Answer from the drawing. Dimensions are ordinates in mm from the lowest x, y and z of the part. Round coordinates to 2 decimals unless told otherwise and drop trailing zeros. Loops run counter-clockwise (first coordinate to the right, second up) from the corner with the lowest first, then second, coordinate; pieces in that order, holes last. Notation, with made-up numbers: M 10.5,-26 L 59.5,-26 A23 cw 59.5,11 Z; hole C 76.25,71.5 d3. An arc over 180 degrees is marked long. Answer as a JSON object with one key per item and string values.
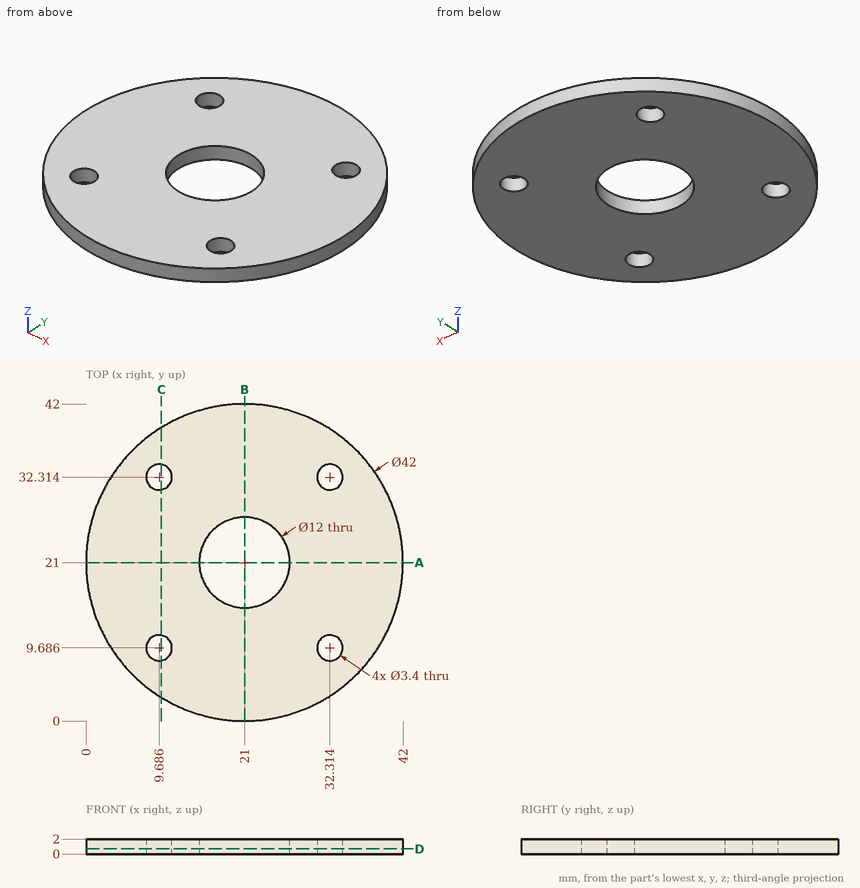
Item 1: The part is cut by section C-C (x = 10). Give the vertices of the cut face in (y, z) (1 decimal).
Values follow:
{"outline": "M 3.1,0 L 8,0 L 8,2 L 3.1,2 Z; M 11.4,0 L 30.6,0 L 30.6,2 L 11.4,2 Z; M 34,0 L 38.9,0 L 38.9,2 L 34,2 Z"}
Item 2: The part is cut by section D-D (z = 0.7). Give the vertices of the cut face in (x, y).
Values follow:
{"outline": "C 21,21 d42; hole C 9.69,9.69 d3.4; hole C 9.69,32.31 d3.4; hole C 21,21 d12; hole C 32.31,9.69 d3.4; hole C 32.31,32.31 d3.4"}
Item 3: Straight lines are drawn through the part: line 1 (Y direction, x = 21, z = 1); line 2 (Y direction, x = 9.5, z = 1.9) (1 decimal); line 3 (Y direction, x = 19, z = 1.6) (1 decimal). For each, find the intervals that lie inside material, in ascending order.
Values follow:
{"line 1": "0 to 15, 27 to 42", "line 2": "3.4 to 8, 11.4 to 30.6, 34 to 38.6", "line 3": "0.1 to 15.3, 26.7 to 41.9"}
Item 4: The part is cut by section A-A (y = 21). Give the vertices of the cut face in (x, z).
Values follow:
{"outline": "M 0,0 L 15,0 L 15,2 L 0,2 Z; M 27,0 L 42,0 L 42,2 L 27,2 Z"}
